```python
from build123d import *

# Parameters (mm, degrees)
SKETCH2_R           = 36.5
BOSS_EXTRUDE1_DEPTH = 2.5
SKETCH3_R           = 36.5
SKETCH3_R_2         = 35
BOSS_EXTRUDE2_DEPTH = 35
SKETCH4_R           = 3.75
BOSS_EXTRUDE3_DEPTH = 35
SKETCH5_R           = 1.225
CUT_EXTRUDE2_DEPTH  = 64.802429421
CUT_EXTRUDE7_START  = -24
CUT_EXTRUDE7_DEPTH  = 24
FILLET2_R           = 0.75
SKETCH17_R          = 4.5
CUT_EXTRUDE9_DEPTH  = 10
SKETCH19_W          = 60.448509469
SKETCH19_H          = 17.659938419
CUT_EXTRUDE10_DEPTH = 10
FILLET7_R           = 1
CUT_EXTRUDE11_START = -12
SKETCH20_R          = 36.5
CUT_EXTRUDE11_DEPTH = 12
SKETCH21_W          = 50.64390868
SKETCH21_H          = 2.55548202
CUT_EXTRUDE13_DEPTH = 3


with BuildPart() as part:
    # Sketch2 → Boss-Extrude1 (new body)
    with BuildSketch(Plane(origin=(0, 0, 0), x_dir=(1, 0, 0), z_dir=(0, 1, 0))):
        with Locations(Location((0, 0, 0), (0, 0, 270))):
            Circle(SKETCH2_R)
    extrude(amount=BOSS_EXTRUDE1_DEPTH)

    # Sketch3 → Boss-Extrude2 (add)
    with BuildSketch(Plane(origin=(0, 2.5, 0), x_dir=(1, 0, 0), z_dir=(0, 1, 0))):
        with Locations(Location((0, 0, 0), (0, 0, 270))):
            Circle(SKETCH3_R)
        with Locations(Location((0, 0, 0), (0, 0, 270))):
            Circle(SKETCH3_R_2, mode=Mode.SUBTRACT)
    extrude(amount=BOSS_EXTRUDE2_DEPTH)

    # Sketch4 → Boss-Extrude3 (add)
    with BuildSketch(Plane(origin=(0, 2.5, 0), x_dir=(1, 0, 0), z_dir=(0, 1, 0))):
        with Locations(Location((-22, 22, 0), (0, 0, 270))):
            Circle(SKETCH4_R)
        with Locations(Location((22, 22, 0), (0, 0, 270))):
            Circle(SKETCH4_R)
        with Locations(Location((22, -22, 0), (0, 0, 270))):
            Circle(SKETCH4_R)
        with Locations(Location((-22, -22, 0), (0, 0, 270))):
            Circle(SKETCH4_R)
    extrude(amount=BOSS_EXTRUDE3_DEPTH)

    # Sketch5 → Cut-Extrude2 (cut, through all)
    with BuildSketch(Plane(origin=(0, 37.5, 0), x_dir=(1, 0, 0), z_dir=(0, 1, 0))):
        with Locations(Location((-22, -22, 0), (0, 0, 270))):
            Circle(SKETCH5_R)
        with Locations(Location((-22.145028028, 22.135381056, 0), (0, 0, 270))):
            Circle(SKETCH5_R)
        with Locations(Location((21.959827612, 22.246616506, 0), (0, 0, 270))):
            Circle(SKETCH5_R)
        with Locations(Location((21.904209888, -21.858239135, 0), (0, 0, 270))):
            Circle(SKETCH5_R)
    extrude(amount=-CUT_EXTRUDE2_DEPTH, mode=Mode.SUBTRACT)

    # Sketch9 → Cut-Extrude7 (cut)
    with BuildSketch(Plane.XZ.offset(CUT_EXTRUDE7_START)):
        with BuildLine():
            ThreePointArc((25.25, 22), (22, 25.25), (18.75, 22))
            Line((18.75, 22), (20.687440042, 22))
            ThreePointArc((20.687440042, 22), (21.975209673, 23.081179865), (23.129209888, 21.858239135))
            ThreePointArc((23.129209888, 21.858239135), (22.803645235, 21.026589536), (22, 20.63699008))
            Line((22, 20.63699008), (22, 18.75))
            ThreePointArc((22, 18.75), (24.298097039, 19.701902961), (25.25, 22))
        make_face()
        with BuildLine():
            Line((20.687440042, 22), (18.75, 22))
            ThreePointArc((18.75, 22), (19.701902961, 19.701902961), (22, 18.75))
            Line((22, 18.75), (22, 20.63699008))
            ThreePointArc((22, 20.63699008), (21.02182794, 21.008517358), (20.687440042, 22))
        make_face()
        with BuildLine():
            ThreePointArc((25.25, -22), (24.298097039, -19.701902961), (22, -18.75))
            Line((22, -18.75), (22, -21.022275385))
            ThreePointArc((22, -21.022275385), (22.840121931, -21.394732175), (23.184827612, -22.246616506))
            ThreePointArc((23.184827612, -22.246616506), (21.835883306, -23.465330093), (20.75990874, -22))
            Line((20.75990874, -22), (18.75, -22))
            ThreePointArc((18.75, -22), (22, -25.25), (25.25, -22))
        make_face()
        with BuildLine():
            Line((22, -21.022275385), (22, -18.75))
            ThreePointArc((22, -18.75), (19.701902961, -19.701902961), (18.75, -22))
            Line((18.75, -22), (20.75990874, -22))
            ThreePointArc((20.75990874, -22), (21.201382273, -21.284646824), (22, -21.022275385))
        make_face()
        with BuildLine():
            ThreePointArc((-18.75, -22), (-19.701902961, -19.701902961), (-22, -18.75))
            Line((-22, -18.75), (-22, -20.918996302))
            ThreePointArc((-22, -20.918996302), (-21.275395744, -21.272615335), (-20.92753184, -22))
            Line((-20.92753184, -22), (-18.75, -22))
        make_face()
        with BuildLine():
            Line((-22, -20.918996302), (-22, -18.75))
            ThreePointArc((-22, -18.75), (-24.298097039, -24.298097039), (-18.75, -22))
            Line((-18.75, -22), (-20.92753184, -22))
            ThreePointArc((-20.92753184, -22), (-20.92190542, -22.067586629), (-20.920028028, -22.135381056))
            ThreePointArc((-20.920028028, -22.135381056), (-23.061075062, -22.948697005), (-22, -20.918996302))
        make_face()
        with BuildLine():
            ThreePointArc((-22, 20.775), (-22.866205807, 22.866205807), (-20.775, 22))
            Line((-20.775, 22), (-18.75, 22))
            ThreePointArc((-18.75, 22), (-24.298097039, 24.298097039), (-22, 18.75))
            Line((-22, 18.75), (-22, 20.775))
        make_face()
        with BuildLine():
            Line((-18.75, 22), (-20.775, 22))
            ThreePointArc((-20.775, 22), (-21.133794193, 21.133794193), (-22, 20.775))
            Line((-22, 20.775), (-22, 18.75))
            ThreePointArc((-22, 18.75), (-19.701902961, 19.701902961), (-18.75, 22))
        make_face()
    extrude(amount=CUT_EXTRUDE7_DEPTH, mode=Mode.SUBTRACT)

    # Fillet2
    fillet2_edges = [part.edges().sort_by_distance(p)[0] for p in [
        (0, 37.5, -35),
    ]]
    fillet(fillet2_edges, radius=FILLET2_R)

    # Sketch17 → Cut-Extrude9 (cut)
    with BuildSketch(Plane.XZ):
        with Locations(Location((0, -26.418957296, 0), (0, 0, 270))):
            Circle(SKETCH17_R)
    extrude(amount=-CUT_EXTRUDE9_DEPTH, mode=Mode.SUBTRACT)

    # Sketch19 → Cut-Extrude10 (cut)
    with BuildSketch(Plane.XZ):
        with Locations((0.023287933, -1.164693847)):
            Rectangle(SKETCH19_W, SKETCH19_H)
    extrude(amount=-CUT_EXTRUDE10_DEPTH, mode=Mode.SUBTRACT)

    # Fillet7
    fillet7_edges = [part.edges().sort_by_distance(p)[0] for p in [
        (0, 0, -36.5),
    ]]
    fillet(fillet7_edges, radius=FILLET7_R)

    # Sketch20 → Cut-Extrude11 (cut)
    with BuildSketch(Plane(origin=(0, 37.5, 0), x_dir=(1, 0, 0), z_dir=(0, 1, 0)).offset(CUT_EXTRUDE11_START)):
        with Locations(Location((0, 0, 0), (0, 0, 270))):
            Circle(SKETCH20_R)
    extrude(amount=CUT_EXTRUDE11_DEPTH, mode=Mode.SUBTRACT)

    # Sketch21 → Cut-Extrude13 (cut)
    with BuildSketch(Plane(origin=(0, 25.5, 0), x_dir=(1, 0, 0), z_dir=(0, 1, 0))):
        with Locations((0, 18.98239711)):
            Rectangle(SKETCH21_W, SKETCH21_H)
    extrude(amount=-CUT_EXTRUDE13_DEPTH, mode=Mode.SUBTRACT)


solid = part.part
```
Check sheet for the modelled part. Datum: model origin and axes. Units: mm. A direction names the side the tool comes from. Coordinates: 2 decimals unless noted, no trailing zeros. Write each loop counter-clockwise with the first axis right and the second up, starting at its lowest first coordinate (ties: lowest second). Pieces come first, ordered by that corner, then holes. Notation, with made-up numbers: (-6.75, 74) - (25.25, 74) arc R12 cw to (25.25, 92) - close; hole circle Ø1 at (39.25, 11.25). An arc over 180 degrees is marked (long way). One line per question, with ' | ' between items.
Item 1: Sectioned sample at B-B on y = 16.5. Give the number of separate pieces and of enclosed holes in the cut face, plus the area to 3 significant figures.
Determined:
separate pieces: 5 | enclosed holes: 5 | area: 381 mm2
Item 2: Mould release check, pull along Z, two halves, no side actions. Record for faces 1 (the face through (22, 24.4, -20.26)), 2 (the face through (0, 0, 15)): pulls with the +Z half, pulls with the -Z half, needs draft (parallel to the pull), parting line crosses it, or undercut.
Determined:
face 1: undercut | face 2: needs draft
Item 3: Gauge pin test, flat ends, axial feed: P1, Ø1, axis at x = -21.5, z = -19, coming from the +Y side; P2, Ø10, axis at x = -14, z = -6, coming from the +Y side; P3, Ø1.5, axis at x = 21, y = 23.5, coming from the +Z side. Record the tip position at first contact, or that the pin passes through.
Determined:
P1: stops at y = 22.5 | P2: stops at y = 2.5 | P3: stops at z = 30.37
Item 4: Sectioned sample at C-C on z = 0. Record the boundary of the cut face in (x, y), plus the area to 3 significant figures.
Determined:
outline: (-36.5, 1) arc R1 ccw to (-35.5, 0) - (-30.2, 0) - (-30.2, 2.5) - (-35, 2.5) - (-35, 25.5) - (-36.5, 25.5) - close; (30.25, 0) - (35.5, 0) arc R1 ccw to (36.5, 1) - (36.5, 25.5) - (35, 25.5) - (35, 2.5) - (30.25, 2.5) - close | area: 99.9 mm2
Item 5: Sectioned sample at A-A on x = 0. Record the boundary of the cut face in (y, z), plus the area to 3 significant figures.
Determined:
outline: (0, -35.5) arc R1 ccw to (1, -36.5) - (25.5, -36.5) - (25.5, -35) - (2.5, -35) - (2.5, -30.92) - (0, -30.92) - close; (0, -21.92) - (2.5, -21.92) - (2.5, -9.99) - (0, -9.99) - close; (0, 7.67) - (2.5, 7.67) - (2.5, 35) - (25.5, 35) - (25.5, 36.5) - (1, 36.5) arc R1 ccw to (0, 35.5) - close | area: 184 mm2
Item 6: Access from +Z, -Z, +X, -X, +Y, -Y to the whole of each face (thin tool, end or side, straight path). Record for faces 3 (the face through (-22, 24.4, -20.26)), 4 (the face through (0, 1, 7.665)), 5 (the face through (-22, 24, 20.6)).
Determined:
face 3: +Y | face 4: +Y, -Y | face 5: -Y
Item 7: Thickness scan on line 1 (X direction, y = 2.75, z = 23.5); line 2 (X direction, y = 17.25, z = 24.5) (1 decimal); line 3 (Z direction, x = -21.5, y = 18.75). Record the ranges inside material, lowest first. Write a range as [from, to].
Determined:
line 1: x = [-27.93, -25.94], [-25.44, -24.88], [-19.12, -18.56], [18.56, 19.12], [24.88, 25.44], [25.94, 27.93] | line 2: x = [-27.1, -25], [-24.8, -24.1], [-19.9, -19.2], [19.2, 19.9], [24.1, 24.8], [25, 27.1] | line 3: z = [-29.5, -27.62], [-25.72, -25.21], [-18.79, -18.28], [18.28, 18.79], [25.21, 25.72], [27.62, 29.5]
